```python
from build123d import *

# Parameters (mm, degrees)
F0_R     = 5
F0_R_2   = 2
F1_DEPTH = 29
F2_DEPTH = 4


with BuildPart() as f1:
    # F0 (on Front) → F1 (new body)
    with BuildSketch(Plane.XZ):
        with Locations((-21.545855, 24.76695)):
            Circle(F0_R)
        with Locations((-21.545855, 24.76695)):
            Circle(F0_R_2, mode=Mode.SUBTRACT)
    extrude(amount=F1_DEPTH)


with BuildPart() as f2:
    # F0 (on Front) → F2 (new body)
    with BuildSketch(Plane.XZ):
        with Locations((-21.545855, 24.76695)):
            Circle(F0_R_2)
    extrude(amount=-F2_DEPTH)


solid = f1.part
```
CAD build for the part. Positions are in the model's coordinates, mm. Round coordinates to 2 decimals unless told otherwise and drop trailing zeros. Loops run counter-clockwise (first coordinate to the right, second up) from the corner with the lowest first, then second, coordinate; pieces in that order, holes last. Notation, with made-up numbers: M 85,20 L 97,20 A24 cw 97,54 Z; hole C 38,79 d2. An arc over 180 degrees is marked long. Use a Markdown table: item, result. Add a question column.
(1) Cut at A-A (x = -21.5). Give the cut face in (y, z).
(2) Pull direction X, two halves, no side cores. Call faces 1 (the face through (-23.02, -14.3, 26.12)), 2 (the face through (-21.6, -29, 22.6)), 3 (the face through (-22.197, -14.297, 29.724)): +X half, -X half, draft (parallel to the pull), parting line (faces both ways), or undercut.
(3) Flat gauge pin, fed straight in: pin 1 (1.5 mm diameter, centred on y = -25, z = 26.5, fed in from -X). Where does the tip first touch, or does it go through?
(4) Drill centre lines: line 1 (X direction, y = -10, z = 24.75); line 2 (Z direction, x = -20.75, y = -24); line 3 (X direction, y = -25, z = 23.5). Where is each one in solid material? Low to high.
(5) Cut at D-D (z = 28). Give the cut face in (x, y), and give its area (3 significant figures).
(6) Cut at B-B (z = 26.25). Give the cut face in (x, y), and give its area (3 significant figures).
(7) Cut at C-C (y = -15). Give the cut face in (x, z), and give its area (3 significant figures).
Geometry says:
| question | item | result |
|---|---|---|
| 1 | outline | M -29,19.77 L 0,19.77 L 0,22.77 L -29,22.77 Z; M -29,26.77 L 0,26.77 L 0,29.77 L -29,29.77 Z |
| 2 | face 1 | undercut |
| 2 | face 2 | draft |
| 2 | face 3 | parting line |
| 3 | pin 1 | stops at x = -26.45 |
| 4 | line 1 | x = -26.55 to -23.55, -19.55 to -16.55 |
| 4 | line 2 | z = 19.83 to 22.93, 26.6 to 29.7 |
| 4 | line 3 | x = -26.38 to -23.09, -20 to -16.71 |
| 5 | outline | M -25.36,-29 L -17.73,-29 L -17.73,0 L -25.36,0 Z |
| 5 | area | 221 mm² |
| 6 | outline | M -26.32,-29 L -22.89,-29 L -22.89,0 L -26.32,0 Z; M -20.2,-29 L -16.77,-29 L -16.77,0 L -20.2,0 Z |
| 6 | area | 199 mm² |
| 7 | outline | C -21.55,24.77 d10; hole C -21.55,24.77 d4 |
| 7 | area | 66.0 mm² |
